Geometry check sheet. Reference: the model listing, model coordinates, mm. Round coordinates to 2 decimals unless told otherwise and drop trailing zeros.
(1) Material ranges on line 1 along Y through (x, z) = (69.5, -2.75); line 2 along Y through (x, z) = (64.5, -0.75), recorded low to high.
(2) Release check for a two-part mould opening along Y. For faces 1 (the face through (-97.15, -96.99, -10.14)), 2 (the face through (-61.111, 22, -10)), 3 (the face through (100, -1, -10)), 4 (the face through (67, -61.111, -10)) record: +Y half, -Y half, draft (parallel to the pull), parting line (faces both ways), or undercut.
(3) Sectioned sample at A-A (x = -21). Give the number of separate pieces and of enclosed holes in the cut face, plus the area to 3 significant figures.
from build123d import *

# Parameters (mm, degrees)
SKETCH1_W                  = 200
SKETCH1_H                  = 200
BOSS_EXTRUDE1_DEPTH        = 20
SKETCH1_3_W                = 11.111111111
SKETCH1_3_H                = 11.111111111
CUT_EXTRUDE2_DEPTH         = 143.828568571
CHAMFER1_SIZE              = 1.333333333
LPATTERN1_COUNT            = 4
LPATTERN1_PITCH            = 44.444444444
LPATTERN1_COUNT_DIR2       = 4
LPATTERN1_PITCH_DIR2       = 44.444444444
CHAMFER1_OF_LPATTERN1_SIZE = 1.333333333
FILLET1_R                  = 10


with BuildPart() as part:
    # Sketch1 → Boss-Extrude1 (new body)
    with BuildSketch(Plane.XY):
        Rectangle(SKETCH1_W, SKETCH1_H)
    extrude(amount=-BOSS_EXTRUDE1_DEPTH)

    # Sketch1_3 → Cut-Extrude2 (cut, symmetric)
    with BuildSketch(Plane.XY):
        with Locations((66.666666667, 66.666666667)):
            Rectangle(SKETCH1_3_W, SKETCH1_3_H)
    cut_extrude2 = extrude(amount=CUT_EXTRUDE2_DEPTH, both=True, mode=Mode.SUBTRACT)

    # Chamfer1
    chamfer1_edges = [part.edges().sort_by_distance(p)[0] for p in [
        (61.111111111, 66.666666667, 0),
        (66.666666667, 61.111111111, 0),
        (72.222222222, 66.666666667, 0),
        (66.666666667, 72.222222222, 0),
        (66.666666667, 72.222222222, -20),
        (61.111111111, 66.666666667, -20),
        (72.222222222, 66.666666667, -20),
        (66.666666667, 61.111111111, -20),
    ]]
    chamfer(chamfer1_edges, length=CHAMFER1_SIZE)

    # LPattern1: Cut-Extrude2 4 × 4
    with Locations(*[(-i * LPATTERN1_PITCH, -j * LPATTERN1_PITCH_DIR2, 0) for i in range(LPATTERN1_COUNT) for j in range(LPATTERN1_COUNT_DIR2) if (i, j) != (0, 0)]):
        add(cut_extrude2, mode=Mode.SUBTRACT)

    # Chamfer1 of LPattern1
    chamfer1_of_lpattern1_edges = [part.edges().sort_by_distance(p)[0] for p in [
        (61.111111111, 22.222222222, 0),
        (66.666666667, 16.666666667, 0),
        (72.222222222, 22.222222222, 0),
        (66.666666667, 27.777777778, 0),
        (66.666666667, 27.777777778, -20),
        (61.111111111, 22.222222222, -20),
        (72.222222222, 22.222222222, -20),
        (66.666666667, 16.666666667, -20),
        (61.111111111, -22.222222222, 0),
        (66.666666667, -27.777777778, 0),
        (72.222222222, -22.222222222, 0),
        (66.666666667, -16.666666667, 0),
        (66.666666667, -16.666666667, -20),
        (61.111111111, -22.222222222, -20),
        (72.222222222, -22.222222222, -20),
        (66.666666667, -27.777777778, -20),
        (61.111111111, -66.666666667, 0),
        (66.666666667, -72.222222222, 0),
        (72.222222222, -66.666666667, 0),
        (66.666666667, -61.111111111, 0),
        (66.666666667, -61.111111111, -20),
        (61.111111111, -66.666666667, -20),
        (72.222222222, -66.666666667, -20),
        (66.666666667, -72.222222222, -20),
        (16.666666667, 66.666666667, 0),
        (22.222222222, 61.111111111, 0),
        (27.777777778, 66.666666667, 0),
        (22.222222222, 72.222222222, 0),
        (22.222222222, 72.222222222, -20),
        (16.666666667, 66.666666667, -20),
        (27.777777778, 66.666666667, -20),
        (22.222222222, 61.111111111, -20),
        (16.666666667, 22.222222222, 0),
        (22.222222222, 16.666666667, 0),
        (27.777777778, 22.222222222, 0),
        (22.222222222, 27.777777778, 0),
        (22.222222222, 27.777777778, -20),
        (16.666666667, 22.222222222, -20),
        (27.777777778, 22.222222222, -20),
        (22.222222222, 16.666666667, -20),
        (16.666666667, -22.222222222, 0),
        (22.222222222, -27.777777778, 0),
        (27.777777778, -22.222222222, 0),
        (22.222222222, -16.666666667, 0),
        (22.222222222, -16.666666667, -20),
        (16.666666667, -22.222222222, -20),
        (27.777777778, -22.222222222, -20),
        (22.222222222, -27.777777778, -20),
        (16.666666667, -66.666666667, 0),
        (22.222222222, -72.222222222, 0),
        (27.777777778, -66.666666667, 0),
        (22.222222222, -61.111111111, 0),
        (22.222222222, -61.111111111, -20),
        (16.666666667, -66.666666667, -20),
        (27.777777778, -66.666666667, -20),
        (22.222222222, -72.222222222, -20),
        (-27.777777778, 66.666666667, 0),
        (-22.222222222, 61.111111111, 0),
        (-16.666666667, 66.666666667, 0),
        (-22.222222222, 72.222222222, 0),
        (-22.222222222, 72.222222222, -20),
        (-27.777777778, 66.666666667, -20),
        (-16.666666667, 66.666666667, -20),
        (-22.222222222, 61.111111111, -20),
        (-27.777777778, 22.222222222, 0),
        (-22.222222222, 16.666666667, 0),
        (-16.666666667, 22.222222222, 0),
        (-22.222222222, 27.777777778, 0),
        (-22.222222222, 27.777777778, -20),
        (-27.777777778, 22.222222222, -20),
        (-16.666666667, 22.222222222, -20),
        (-22.222222222, 16.666666667, -20),
        (-27.777777778, -22.222222222, 0),
        (-22.222222222, -27.777777778, 0),
        (-16.666666667, -22.222222222, 0),
        (-22.222222222, -16.666666667, 0),
        (-22.222222222, -16.666666667, -20),
        (-27.777777778, -22.222222222, -20),
        (-16.666666667, -22.222222222, -20),
        (-22.222222222, -27.777777778, -20),
        (-27.777777778, -66.666666667, 0),
        (-22.222222222, -72.222222222, 0),
        (-16.666666667, -66.666666667, 0),
        (-22.222222222, -61.111111111, 0),
        (-22.222222222, -61.111111111, -20),
        (-27.777777778, -66.666666667, -20),
        (-16.666666667, -66.666666667, -20),
        (-22.222222222, -72.222222222, -20),
        (-72.222222222, 66.666666667, 0),
        (-66.666666667, 61.111111111, 0),
        (-61.111111111, 66.666666667, 0),
        (-66.666666667, 72.222222222, 0),
        (-66.666666667, 72.222222222, -20),
        (-72.222222222, 66.666666667, -20),
        (-61.111111111, 66.666666667, -20),
        (-66.666666667, 61.111111111, -20),
        (-72.222222222, 22.222222222, 0),
        (-66.666666667, 16.666666667, 0),
        (-61.111111111, 22.222222222, 0),
        (-66.666666667, 27.777777778, 0),
        (-66.666666667, 27.777777778, -20),
        (-72.222222222, 22.222222222, -20),
        (-61.111111111, 22.222222222, -20),
        (-66.666666667, 16.666666667, -20),
        (-72.222222222, -22.222222222, 0),
        (-66.666666667, -27.777777778, 0),
        (-61.111111111, -22.222222222, 0),
        (-66.666666667, -16.666666667, 0),
        (-66.666666667, -16.666666667, -20),
        (-72.222222222, -22.222222222, -20),
        (-61.111111111, -22.222222222, -20),
        (-66.666666667, -27.777777778, -20),
        (-72.222222222, -66.666666667, 0),
        (-66.666666667, -72.222222222, 0),
        (-61.111111111, -66.666666667, 0),
        (-66.666666667, -61.111111111, 0),
        (-66.666666667, -61.111111111, -20),
        (-72.222222222, -66.666666667, -20),
        (-61.111111111, -66.666666667, -20),
        (-66.666666667, -72.222222222, -20),
    ]]
    chamfer(chamfer1_of_lpattern1_edges, length=CHAMFER1_OF_LPATTERN1_SIZE)

    # Fillet1
    fillet1_edges = [part.edges().sort_by_distance(p)[0] for p in [
        (-100, -100, -10),
        (100, -100, -10),
        (100, 100, -10),
        (-100, 100, -10),
    ]]
    fillet(fillet1_edges, radius=FILLET1_R)


solid = part.part
Answer below:
1. line 1: y = -100 to -72.22, -61.11 to -27.78, -16.67 to 16.67, 27.78 to 61.11, 72.22 to 100
1. line 2: y = -100 to -72.81, -60.53 to -28.36, -16.08 to 16.08, 28.36 to 60.53, 72.81 to 100
2. face 1: -Y half
2. face 2: undercut
2. face 3: draft
2. face 4: undercut
3. separate pieces: 5
3. enclosed holes: 0
3. area: 3,100 mm2
